Here's how the part is built. I have some questions about the finished solid (model axes, mm). A direction names the side the tool comes from. Coordinates: 2 decimals unless noted, no trailing zeros. Order: outer loops, then holes, each group sorted by start corner. A loop starts at its lowest first (then second) coordinate and runs counter-clockwise, first axis right, second up. Notation, with made-up numbers: M 23.5,33 L 34.5,33 A14 cw 34.5,53 Z; hole C -15,73 d5. An arc over 180 degrees is marked long. One line per question, with ' | ' between items. Start each with the question number.
```python
from build123d import *

# Parameters (mm, degrees)
F5_R      = 37
F5_R_2    = 35.5
F6_DEPTH  = 10
F7_R      = 37
F7_R_2    = 32.5
F8_DEPTH  = 5
F4_W      = 20
F4_H      = 50
F9_DEPTH  = 5.5
F11_DEPTH = 10


with BuildPart() as f2:
    # F1 (on Front) → F2 (revolve)
    with BuildSketch(Plane.XZ):
        with BuildLine():
            Line((-37, 0), (0, 0))
            Line((0, 0), (0, 16.45))
            ThreePointArc((0, 16.45), (-20.2460026919, 12.152179307), (-37, 0))
        make_face()
    revolve(axis=Axis((0, 0, 8.225), (0, 0, 1)))

    # F5 (on Top) → F6 (join)
    with BuildSketch(Plane.XY):
        Circle(F5_R)
        Circle(F5_R_2, mode=Mode.SUBTRACT)
    extrude(amount=-F6_DEPTH)

    # F7 (on face) → F8 (join)
    with BuildSketch(Plane(origin=(0, 0, -10), x_dir=(1, 0, 0), z_dir=(0, 0, -1))):
        Circle(F7_R)
        Circle(F7_R_2, mode=Mode.SUBTRACT)
    extrude(amount=F8_DEPTH)

    # F4 (on offset) → F9 (cut)
    with BuildSketch(Plane.XY.offset(16.45)):
        with Locations((-15, 0)):
            Rectangle(F4_W, F4_H)
        with Locations((15, 0)):
            Rectangle(F4_W, F4_H)
    extrude(amount=-F9_DEPTH, mode=Mode.SUBTRACT)

    # F10 (on face) → F11 (cut)
    with BuildSketch(Plane(origin=(0, 0, -15), x_dir=(1, 0, 0), z_dir=(0, 0, -1))):
        with BuildLine():
            ThreePointArc((-31.0352267718, -9.6470046761), (-32.4780480974, -1.1943164501), (-31.6599461457, 7.3415127902))
            Line((-31.6599461457, 7.3415127902), (-34.6599461457, 7.3415127902))
            ThreePointArc((-34.6599461457, 7.3415127902), (-35.4051205032, -1.298891462), (-34.0288283151, -9.8614664413))
            Line((-34.0288283151, -9.8614664413), (-31.0352267718, -9.6470046761))
        make_face()
        with BuildLine():
            ThreePointArc((9.6470046761, -31.0352267718), (1.1943164501, -32.4780480974), (-7.3415127902, -31.6599461457))
            Line((-7.3415127902, -31.6599461457), (-7.3415127902, -34.6599461457))
            ThreePointArc((-7.3415127902, -34.6599461457), (1.298891462, -35.4051205032), (9.8614664413, -34.0288283151))
            Line((9.8614664413, -34.0288283151), (9.6470046761, -31.0352267718))
        make_face()
        with BuildLine():
            Line((34.0288283151, 9.8614664413), (31.0352267718, 9.6470046761))
            ThreePointArc((31.0352267718, 9.6470046761), (32.131720076, 4.8787872425), (32.5, 0))
            ThreePointArc((32.5, 0), (32.2893035674, -3.6947090727), (31.6599461457, -7.3415127902))
            Line((31.6599461457, -7.3415127902), (34.6599461457, -7.3415127902))
            ThreePointArc((34.6599461457, -7.3415127902), (35.4051205032, 1.298891462), (34.0288283151, 9.8614664413))
        make_face()
        with BuildLine():
            Line((-9.8614664413, 34.0288283151), (-9.6470046761, 31.0352267718))
            ThreePointArc((-9.6470046761, 31.0352267718), (-1.1943164501, 32.4780480974), (7.3415127902, 31.6599461457))
            Line((7.3415127902, 31.6599461457), (7.3415127902, 34.6599461457))
            ThreePointArc((7.3415127902, 34.6599461457), (-1.298891462, 35.4051205032), (-9.8614664413, 34.0288283151))
        make_face()
    extrude(amount=-F11_DEPTH, mode=Mode.SUBTRACT)


solid = f2.part
```
1. Imagine slicing it at D-D (y = -20). List the corners of the cut face in (x, z) for me.
2. Imagine slicing it at B-B (y = 0). List the corners of the cut face in (x, z) for me, then the cut area to 3 significant figures.
3. Imagine slicing it at A-A (x = 0). List the corners of the cut face in (y, z) for me, then the cut area to 3 significant figures.
4. I need wall thicknesses on line 1 (Y direction, x = 0, z = -5); line 2 (Y direction, x = 30.5, z = -7.5); line 3 (Z direction, x = 22, y = 4). Which ranges of each line are inside material? Lowest first, please.
5. Which directions (+Z, -Z, +X, -X, +Y, -Y) give clear straight access to the entire face, cutting with the end or side of a thin tool? Please do faces 1 (the face through (0, 0, 0)), 2 (the face through (-12, 0, 10.95)), 3 (the face through (33, 7.342, -13)).
6. Will these pins go through, and if not, where does the flat tip stop? pin 1 (1.5 mm diameter, centred on x = -11.5, z = -10, fed in from -Y); pin 2 (3.5 mm diameter, centred on y = -33.5, z = -12.5, fed in from -X); pin 3 (8 mm diameter, centred on y = -17, z = -6, fed in from +X).
7. We'd pull the mould along Y, two halves only. Please class faces 4 (the face through (5, 0, 13)), 5 (the face through (-32.553, 9.756, -12.535)): released by +Y, released by -Y, zero draft, split by the parting line, or undercut.
8. Imagine slicing it at C-C (z = 14.5). List the corners of the cut face in (x, y) for me, then the cut area to 3 significant figures.
Entries:
1) outline: M -31.13,-15 L -25.62,-15 L -25.62,-10 L -29.33,-10 L -29.33,0 L 29.33,0 L 29.33,-10 L 25.62,-10 L 25.62,-15 L 31.13,-15 L 31.13,0 A45.65 ccw 10.86,10.95 L 5,10.95 L 5,11.99 A45.65 ccw -5,11.99 L -5,10.95 L -10.86,10.95 A45.65 ccw -31.13,0 Z
2) outline: M -37,-15 L -35.43,-15 L -35.43,-10 L -35.5,-10 L -35.5,0 L 35.5,0 L 35.5,-10 L 35.43,-10 L 35.43,-15 L 37,-15 L 37,0 A49.84 ccw 22.76,10.95 L 5,10.95 L 5,16.2 A49.84 ccw -5,16.2 L -5,10.95 L -22.76,10.95 A49.84 ccw -37,0 Z | area: 774 mm²
3) outline: M -37,-15 L -35.43,-15 L -35.43,-10 L -35.5,-10 L -35.5,0 L 35.5,0 L 35.5,-10 L 35.43,-10 L 35.43,-15 L 37,-15 L 37,0 A49.84 ccw -37,0 Z | area: 888 mm²
4) line 1: -37 to -35.5, 35.5 to 37 | line 2: -20.95 to -18.17, 18.17 to 20.95 | line 3: 0 to 10.95
5) face 1: none | face 2: +Z, -X, +Y, -Y | face 3: -Z
6) pin 1: y = -35.4 | pin 2: x = -19 | pin 3: x = 34.64
7) face 4: zero draft | face 5: undercut
8) outline: M -5,-12.87 A13.8 ccw 5,-12.87 L 5,12.87 A13.8 ccw -5,12.87 Z | area: 270 mm²
